For this review, take the finished solid that the model builds, in its own axes (mm). Face numbers are marked on the shaded views. Round coordinates to 2 decimals unless told otherwise and drop trailing zeros. Write each loop counter-clockwise with the first axis right and the second up, starting at its lowest first coordinate (ties: lowest second). Pieces come first, ordered by that corner, then holes. Notation, with made-up numbers: (-23, 73.25) -> (26, 73.25) arc R23 cw to (26, 91.25) -> close; hole circle Ø1 at (10.25, -5). An arc over 180 degrees is marked (long way). Answer as CSV lines item,"result". Start each with the question number.
Item 1: Take a section at C-C on z = 2.05. Give the boundary of the cut face in (x, y), then the cut area to 3 significant figures.
Item 2: Take a section at B-B on x = 0. Give the boundary of the cut face in (y, z), then the cut area to 3 significant figures.
Item 3: Wall thickness on probe 1 along Y at (x, z) = (0, 3.8); probe 2 along X at (y, z) = (-12.25, 4.2); probe 3 along X at (y, z) = (-0.25, 2.25): over which ranges is each line inside the solid? List them lowest first. Write a range as from..to.
Item 4: Take a section at A-A on y = 0. Give the boundary of the cut face in (x, z).
Item 5: Take a section at D-D on x = -24. Give the boundary of the cut face in (y, z).
Item 6: Mouldability with a two-part tool opening along Y and no side actions: class the marked faces 1, 2, 3 and 4 as +Y half, -Y half, draft (parallel to the pull), parting line (faces both ways), or undercut.
Item 7: For pin 1 Ø1 at (x, z) = (-32.5, 3) entering from +Y; pin 2 Ø2.5 at (x, z) = (-20.5, 3.5) entering from -Y; pin 3 Ø1 at (x, z) = (-13.5, 0.5) entering from -Y, all flat-tipped, find the tip position at first contact; note any pin that passes through.
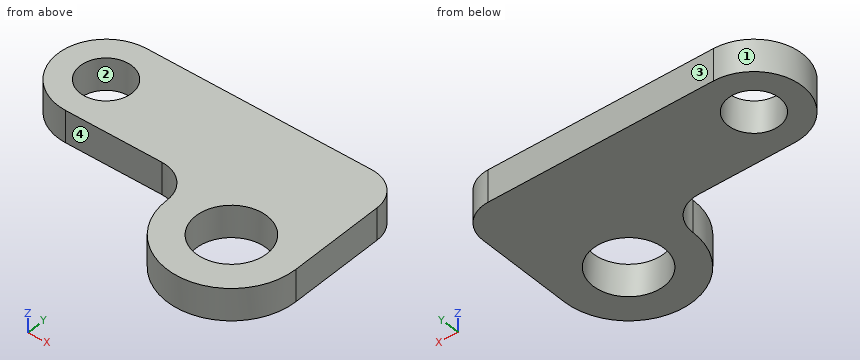
```python
from build123d import *

# Parameters (mm, degrees)
SKETCH_1_R       = 4
SKETCH_1_R_2     = 5.5
EXTRUDE_1_DEPTH  = 5
FILLET_1_DEPTH   = 5
FILLET_1_2_DEPTH = 5


with BuildPart() as part:
    # 草图1 → 凸台-拉伸1 (new body)
    with BuildSketch(Plane.XY):
        with BuildLine():
            Line((-30, -7.5), (-10, -7.5))
            Line((-10, -7.5), (-10, -12.5))
            ThreePointArc((-10, -12.5), (0, -22.5), (10, -12.5))
            Line((10, -12.5), (10, 7.5))
            Line((10, 7.5), (-30, 7.5))
            ThreePointArc((-30, 7.5), (-37.5, 0), (-30, -7.5))
        make_face()
        with Locations((-30, 0)):
            Circle(SKETCH_1_R, mode=Mode.SUBTRACT)
        with Locations((0, -12.5)):
            Circle(SKETCH_1_R_2, mode=Mode.SUBTRACT)
    extrude(amount=EXTRUDE_1_DEPTH)

    # 圆角1: read off the stored shape, not the designer's step
    # 圆角1 outline → 圆角1 (cut)
    with BuildSketch(Plane.XY):
        with BuildLine():
            Line((10, 7.5), (5, 7.5))
            ThreePointArc((5, 7.5), (8.535533906, 6.035533906), (10, 2.5))
            Line((10, 2.5), (10, 7.5))
        make_face()
    extrude(amount=FILLET_1_DEPTH, mode=Mode.SUBTRACT)

    # Fillet 1 2 outline → Fillet 1 2 (add)
    with BuildSketch(Plane.XY):
        with BuildLine():
            ThreePointArc((-15, -7.5), (-11.464466094, -8.964466094), (-10, -12.5))
            Line((-10, -12.5), (-10, -7.5))
            Line((-10, -7.5), (-15, -7.5))
        make_face()
    extrude(amount=FILLET_1_2_DEPTH)


solid = part.part
```
Output values:
1,outline,"(-30, -7.5) -> (-15, -7.5) arc R5 cw to (-10, -12.5) arc R10 ccw to (10, -12.5) -> (10, 2.5) arc R5 ccw to (5, 7.5) -> (-30, 7.5) arc R7.5 ccw to start; hole circle Ø8 at (-30, 0); hole circle Ø11 at (0, -12.5)"
1,area,"800 mm^2"
2,outline,"(-22.5, 0) -> (-18, 0) -> (-18, 5) -> (-22.5, 5) -> close; (-7, 0) -> (7.5, 0) -> (7.5, 5) -> (-7, 5) -> close"
2,area,"95.0 mm^2"
3,probe 1,"y = -22.5..-18, -7..7.5"
3,probe 2,"x = -10.01..-5.49, 5.49..10"
3,probe 3,"x = -37.5..-33.99, -26.01..10"
4,outline,"(-37.5, 0) -> (-34, 0) -> (-34, 5) -> (-37.5, 5) -> close; (-26, 0) -> (10, 0) -> (10, 5) -> (-26, 5) -> close"
5,outline,"(-7.5, 0) -> (7.5, 0) -> (7.5, 5) -> (-7.5, 5) -> close"
6,face 1,"parting line"
6,face 2,"undercut"
6,face 3,"+Y half"
6,face 4,"-Y half"
7,pin 1,"stops at y = 7.23"
7,pin 2,"stops at y = -7.5"
7,pin 3,"stops at y = -7.92"
